from build123d import *

# Parameters (mm, degrees)
SKETCH1_R      = 2.3876
EXTRUDE1_DEPTH = 9.525


with BuildPart() as part:
    # Sketch1 → Extrude1 (new body)
    with BuildSketch(Plane(origin=(0, 0, 0), x_dir=(1, 0, 0), z_dir=(0, 1, 0))):
        with BuildLine():
            Line((-38.1, 38.1), (-38.1, -152.4))
            Line((-38.1, -152.4), (38.1, -152.4))
            Line((38.1, -152.4), (38.1, -6.35))
            Line((38.1, -6.35), (27.86051193, -6.35))
            ThreePointArc((27.86051193, -6.35), (-14.509197932, -24.617347549), (-19.05, 21.298547486))
            Line((-19.05, 21.298547486), (-19.05, 38.1))
            Line((-19.05, 38.1), (-38.1, 38.1))
        make_face()
        with Locations(Location((-28.575, 28.575, 0), (0, 0, 270))):
            Circle(SKETCH1_R, mode=Mode.SUBTRACT)
        with Locations(Location((28.575, -28.575, 0), (0, 0, 270))):
            Circle(SKETCH1_R, mode=Mode.SUBTRACT)
        with Locations(Location((-28.575, -28.575, 0), (0, 0, 270))):
            Circle(SKETCH1_R, mode=Mode.SUBTRACT)
    extrude(amount=-EXTRUDE1_DEPTH)


solid = part.part
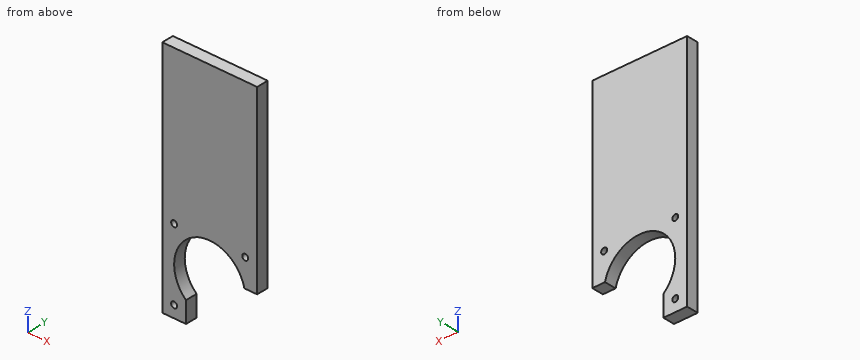
Here's how the part is built. I have some questions about the finished solid (model axes, mm). Coordinates: 2 decimals unless noted, no trailing zeros. Order: outer loops, then holes, each group sorted by start corner. A loop starts at its lowest first (then second) coordinate and runs counter-clockwise, first axis right, second up. Notation, with made-up numbers: M 38.5,41 L 75.5,41 A32 cw 75.5,79 Z; hole C -21,43.25 d6. An arc over 180 degrees is marked long. Answer as CSV lines item,"result". Start each with the question number.
1. I want a section at A-A, the plane y = -2.5. Write out the boundary of the cut face in (x, z) (3 decimals).
2. I want a section at B-B, the plane z = 12.5. Write out the boundary of the cut face in (x, y) (3 decimals), and give its area (3 significant figures).
3. For pin 1 (2 mm diameter, centred on x = -10.5, y = -4.5, fed in from -Z); pin 2 (4.5 mm diameter, centred on x = 28.575, z = 28.575, fed in from -Y); pin 3 (3 mm diameter, centred on x = 34.5, y = -6.5, fed in from -Z); pin 4 (3 mm diameter, centred on y = -4.5, z = -28, fed in from +X), each with a flat end and sliding along its axis, tell me the tip position at first contact or that it passes through.
4. I need wall thicknesses on line 1 (Z direction, x = 34, y = -5); line 2 (X direction, y = -5.25, z = 0) (3 decimals); line 3 (X direction, y = -1.75, z = 11). Which ranges of each line are inside material? Lowest first, please. Write a range as [from, to].
5. I want a section at D-D, the plane x = 10. Write out the boundary of the cut face in (y, z) (3 decimals).
6. I want a section at C-C, the plane x = 0. Write out the boundary of the cut face in (y, z) (3 decimals).
Recorded:
1,outline,"M -38.1,-38.1 L -19.05,-38.1 L -19.05,-21.299 A28.575 cw long 27.861,6.35 L 38.1,6.35 L 38.1,152.4 L -38.1,152.4 Z; hole C -28.575,-28.575 d4.775; hole C -28.575,28.575 d4.775; hole C 28.575,28.575 d4.775"
2,outline,"M -38.1,-9.525 L -25.696,-9.525 L -25.696,0 L -38.1,0 Z; M 25.696,-9.525 L 38.1,-9.525 L 38.1,0 L 25.696,0 Z"
2,area,"236 mm2"
3,pin 1,"stops at z = 26.16"
3,pin 2,"passes through"
3,pin 3,"stops at z = 6.35"
3,pin 4,"stops at x = -19.05"
4,line 1,"z = [6.35, 152.4]"
4,line 2,"x = [-38.1, -28.575]"
4,line 3,"x = [-38.1, -26.37], [26.37, 38.1]"
5,outline,"M -9.525,26.768 L 0,26.768 L 0,152.4 L -9.525,152.4 Z"
6,outline,"M -9.525,28.575 L 0,28.575 L 0,152.4 L -9.525,152.4 Z"
